For this review, take the finished solid that the model builds, in its own axes (mm). A direction names the side the tool comes from. Coordinates: 2 decimals unless noted, no trailing zeros. Write each loop counter-clockwise with the first axis right and the second up, starting at its lowest first coordinate (ties: lowest second). Pieces come first, ordered by that corner, then holes. Notation, with made-up numbers: (87.5, 29) - (94.5, 29) arc R10 cw to (94.5, 42) - close; hole circle Ø6 at (-20.75, 88). An arc over 180 degrees is marked (long way). Use one line per item in the form item = value. Start each with the question number.
1) Tool access review of faces 1 (the flat face through (6.35, 3, -63)), 2 (the flat face through (-63, 3, -6.35)), 3 (the flat face through (63, 3, -6.35)): name each direction out of +Z, -Z, +X, -X, +Y, -Y from which nothing blocks a thin tool from reaching the whole face with its end or side.
2) For L1, parallel to X at y = 4.7, z = 1.5; L2, parallel to X at y = 4.35, z = -35.5; L3, parallel to Z at x = -44, y = 2.35, list the stretches that pass through material, from the lowest coordinate up. Write a range as from..to.
3) We need section A-A (y = 2.6). Give the boundary of the cut face in (x, z).
4) Mouldability with a two-part tool opening along Z and no side actions: class faces 4 (the flat face through (-6.35, 3, 63)), 5 (the flat face through (63, 3, 6.35)), 6 (the flat face through (0, 3, 60.96)) as pulls with the +Z half, pulls with the -Z half, needs draft (parallel to the pull), parting line crosses it, or undercut.
5) Insertion check: P1, Ø3, axis at y = 3, z = 15.5, coming from the +X side; P2, Ø3, axis at y = 2.5, z = 38.5, coming from the -X side; P3, Ø1.5, axis at x = -35.5, z = 51.5, coming from the -Y side; P4, Ø1.5, axis at y = 1.5, z = -3, coming from the +X side. Each pin has a flat end and moves straight along its axis. Give the tip position at first contact, or say it passes through.
6) We need section B-B (x = 4.5). Give the boundary of the cut face in (y, z).
7) We need section C-C (z = -3.5). Give the boundary of the cut face in (x, y).
```python
from build123d import *

# Parameters (mm, degrees)
SKETCH2_R           = 64.77
BOSS_EXTRUDE1_DEPTH = 5.08
FILLET1_R           = 0.635
SKETCH3_W           = 12.7
SKETCH3_H           = 15.225369524
SKETCH3_W_2         = 15.225369524
SKETCH3_H_2         = 12.7
CUT_EXTRUDE1_DEPTH  = 92.739371117


with BuildPart() as part:
    # Sketch2 → Boss-Extrude1 (new body)
    with BuildSketch(Plane(origin=(0, 0, 0), x_dir=(1, 0, 0), z_dir=(0, 1, 0))):
        with Locations(Location((0, 0, 0), (0, 0, 270))):
            Circle(SKETCH2_R)
    extrude(amount=BOSS_EXTRUDE1_DEPTH)

    # Fillet1
    fillet1_edges = [part.edges().sort_by_distance(p)[0] for p in [
        (0, 0, -64.77),
        (0, 5.08, -64.77),
    ]]
    fillet(fillet1_edges, radius=FILLET1_R)

    # Sketch3 → Cut-Extrude1 (cut, through all)
    with BuildSketch(Plane.XZ):
        with Locations((0, 68.572684762)):
            Rectangle(SKETCH3_W, SKETCH3_H)
        with Locations((68.572684762, 0)):
            Rectangle(SKETCH3_W_2, SKETCH3_H_2)
        with Locations((0, -68.572684762)):
            Rectangle(SKETCH3_W, SKETCH3_H)
        with Locations((-68.572684762, 0)):
            Rectangle(SKETCH3_W_2, SKETCH3_H_2)
    extrude(amount=-CUT_EXTRUDE1_DEPTH, mode=Mode.SUBTRACT)


solid = part.part
```
Determined:
q1.face_1 = -Z, +Y, -Y
q1.face_2 = -X, +Y, -Y
q1.face_3 = +X, +Y, -Y
q2.L1 = -60.96..60.96
q2.L2 = -54.17..54.17
q2.L3 = -47.53..47.53
q3.outline = (-64.46, -6.35) arc R64.77 ccw to (-6.35, -64.46) - (-6.35, -60.96) - (6.35, -60.96) - (6.35, -64.46) arc R64.77 ccw to (64.46, -6.35) - (60.96, -6.35) - (60.96, 6.35) - (64.46, 6.35) arc R64.77 ccw to (6.35, 64.46) - (6.35, 60.96) - (-6.35, 60.96) - (-6.35, 64.46) arc R64.77 ccw to (-64.46, 6.35) - (-60.96, 6.35) - (-60.96, -6.35) - close
q4.face_4 = needs draft
q4.face_5 = undercut
q4.face_6 = pulls with the +Z half
q5.P1 = 63.24
q5.P2 = -53.16
q5.P3 = 0
q5.P4 = 60.96
q6.outline = (0, -60.96) - (5.08, -60.96) - (5.08, 60.96) - (0, 60.96) - close
q7.outline = (-60.96, 0) - (60.96, 0) - (60.96, 5.08) - (-60.96, 5.08) - close
